Autodesk Inventor part; units mm, degrees
ref_plane "YZ Plane" through (0, 0, 0) normal (1, 0, 0) x (0, 1, 0)
ref_plane "XZ Plane" through (0, 0, 0) normal (0, 1, 0) x (-1, 0, 0)
ref_plane "XY Plane" through (0, 0, 0) normal (0, 0, 1) x (1, 0, 0)
sketch "Эскиз2" plane through (0, 0, 0) normal (0, 0, 1) x (1, 0, 0)
  line L0 (0, 0) -> (12.5, 0)
  line L1 (12.5, 0) -> (12.5, 22.4)
  line L2 (12.5, 22.4) -> (0, 22.4)
  line L3 (0, 22.4) -> (0, 0)
  dimension "d0" = 12.5
  dimension "d1" = 22.4
extrude "Выдавливание1" add sketch "Эскиз2" along normal blind 22.8
sketch "Эскиз3" plane through (0, 22.4, 0) normal (0, 1, 0) x (1, 0, 0)
  line L0 (12.5, 0) -> (0, 0)
  line L1 (12.5, 0) -> (12.5, -18.1)
  line L2 (12.5, 0) -> (12.5, -22.8)
  line L3 (0, 0) -> (0, -22.8)
  line L4 (12.5, -18.1) -> (0, -18.1)
  line L5 (0, -18.1) -> (0, -21.1)
  line L6 (0, -21.1) -> (12.5, -21.1)
  line L7 (12.5, -21.1) -> (12.5, -18.1)
  point P0 (12.5, -21.1)
  point P1 (0, -18.1)
  dimension "d4" = 18.1
  dimension "d5" = 3
extrude "Выдавливание2" add sketch "Эскиз3" along normal blind 4.7 contours L2 L6 L3 L4
sketch "Эскиз4" plane through (0, 0, 0) normal (0, -1, 0) x (1, 0, 0)
  line L0 (12.2114, 0) -> (12.5, 16.0974)
  line L1 (12.5, 0) -> (12.5, 22.8)
  line L2 (12.5, 21.1) -> (12.5, 18.1)
  line L3 (0, 18.1) -> (0, 21.1)
  line L4 (12.5, 18.1) -> (0, 18.1)
  line L5 (0, 18.1) -> (0, 21.1)
  line L6 (0, 21.1) -> (12.5, 21.1)
  line L7 (12.5, 21.1) -> (12.5, 18.1)
  point P0 (0, 0)
  point P1 (12.5, 21.1)
  point P2 (0, 18.1)
  dimension "d8" = 16.1
  dimension "d9" = 3
extrude "Выдавливание3" add sketch "Эскиз4" along normal blind 4.7
sketch "Эскиз5" plane through (0, 0, 21.1) normal (0, 0, 1) x (1, 0, 0)
  line L0 (0, -4.7) -> (12.5, -4.7)
  line L1 (6.25, -4.7) -> (6.25, -2.275)
  line L2 (12.5, 27.1) -> (0, 27.1)
  line L3 (6.25, 27.1) -> (6.25, 24.675)
  circle A0 centre (6.25, -2.275) radius 1
  circle A1 centre (6.25, 24.675) radius 1
  line L4 (6.25, -2.275) -> (7, -2.275)
  line L5 (7, -2.275) -> (7, -4.7)
  line L6 (7, -4.7) -> (6.25, -4.7)
  line L7 (6.25, -4.7) -> (6.25, -2.275)
  line L8 (6.25, -4.7) -> (5.5, -4.7)
  line L9 (5.5, -4.7) -> (5.5, -2.275)
  line L10 (5.5, -2.275) -> (6.25, -2.275)
  line L11 (6.25, -2.275) -> (6.25, -4.7)
  line L12 (6.25, 27.1) -> (7, 27.1)
  line L13 (7, 27.1) -> (7, 24.675)
  line L14 (7, 24.675) -> (6.25, 24.675)
  line L15 (6.25, 24.675) -> (6.25, 27.1)
  line L16 (6.25, 24.675) -> (5.5, 24.675)
  line L17 (5.5, 24.675) -> (5.5, 27.1)
  line L18 (5.5, 27.1) -> (6.25, 27.1)
  line L19 (6.25, 27.1) -> (6.25, 24.675)
  point P0 (0, 0)
  point P1 (5.5, 25.3364)
  point P2 (7, 25.3364)
  point P3 (5.5, -2.9364)
  point P4 (7, -2.9364)
  dimension "d12" = 2.425
  dimension "d13" = 2.425
  dimension "d14" = 2
  dimension "d15" = 2
  dimension "d16" = 0.75
  dimension "d17" = 0.75
  dimension "d18" = 0.75
  dimension "d19" = 0.75
extrude "Выдавливание4" cut sketch "Эскиз5" against normal through all
sketch "Эскиз6" plane through (0, 0, 22.8) normal (0, 0, 1) x (1, 0, 0)
  line L0 (12.5, 0) -> (0, 0)
  line L1 (6.25, 0) -> (6.25, 6.25)
  circle A0 centre (6.25, 6.25) radius 6.25
  line L2 (6.25, 6.25) -> (6.25, 13.5)
  circle A1 centre (6.25, 13.5) radius 2
  point P0 (7.8448, 12.2931)
  dimension "d22" = 6.25
  dimension "d23" = 12.5
  dimension "d24" = 7.25
  dimension "d25" = 4
extrude "Выдавливание5" add sketch "Эскиз6" along normal blind 5
sketch "Эскиз7" plane through (0, 0, 27.8) normal (0, 0, 1) x (1, 0, 0)
  arc A0 (4.6552, 12.2931) -> (0, 6.25) centre (6.25, 6.25) ccw
  circle A1 centre (6.25, 6.25) radius 1.5
  point P0 (0, 0)
  dimension "d28" = 3
extrude "Выдавливание6" add sketch "Эскиз7" along normal blind 4.6
properties part number "Сервопривод SG90"
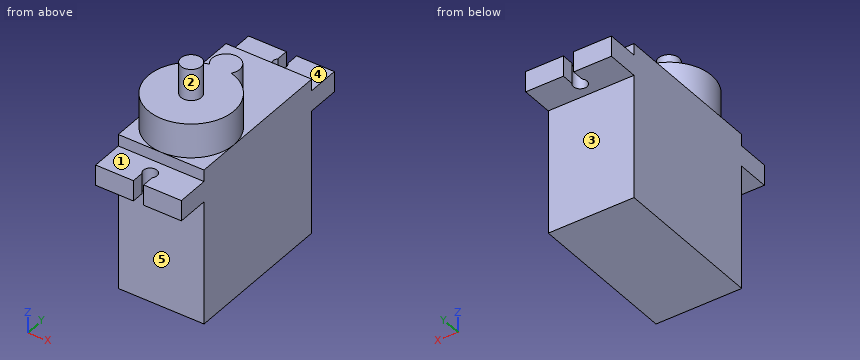
Check sheet for the modelled part. Datum: model origin and axes. Units: mm. Face numbers are marked on the shaded views. A direction names the side the tool comes from. Give positions to 0.01 mm unless a question says otherwise; leave off trailing zeros. Write each loop counter-clockwise with the first axis right and the second up, starting at its lowest first coordinate (ties: lowest second). Pieces come first, ordered by that corner, then holes. Notation, with made-up numbers: (27, 16.5) -> (56, 16.5) arc R25 cw to (56, 30.5) -> close; hole circle Ø5 at (16, -16). An arc over 180 degrees is marked (long way). One line per item, written item: value. Start each with the question number.
Item 1: Tool access check on the marked faces 1, 2, 3, 4 and 5. Record the directions out of +Z, -Z, +X, -X, +Y, -Y that give a thin tool (end or side, any length) a straight path to the whole face; none if there is none.
Item 2: Gauge pin test, flat ends, axial feed: pin 1 (6 mm diameter, centred on x = 4.5, z = 3.5, fed in from +Y); pin 2 (1 mm diameter, centred on x = 7, y = 14, fed in from +Z); pin 3 (3 mm diameter, centred on x = 6.25, y = -2.275, fed in from -Z). Record the tip position at first contact, or that the pin passes through.
Item 3: Material ranges on probe 1 along Y at (x, z) = (2.25, 14); probe 2 along Y at (x, z) = (6.25, 18.9) (3 decimals); probe 3 along Z at (x, y) = (3.75, 25), recorded low to high. Write a range as from..to.
Item 4: Section check D-D on y = 4. Record the cut outline in (x, z).
Item 5: Section check A-A on y = 13.5. Record the cut outline in (x, z), then the cut area to 3 significant figures.
Item 6: Section check C-C on z = 6. Record the cut outline in (x, y).
Item 7: Section check B-B on x = 9. Record the cut outline in (y, z), then the cut area to 3 significant figures.
Results list:
1. face 1: +Z, +X, -X, -Y
1. face 2: +Z
1. face 3: -Z, +X, -X, +Y
1. face 4: +Z, +X, -X, +Y
1. face 5: -Z, +X, -X, -Y
2. pin 1: y = 22.4
2. pin 2: z = 27.8
2. pin 3: z = 18.1
3. probe 1: 0..22.4
3. probe 2: -1.275..23.675
3. probe 3: 18.1..21.1
4. outline: (0, 0) -> (12.5, 0) -> (12.5, 22.8) -> (12.08, 22.8) -> (12.08, 27.8) -> (0.42, 27.8) -> (0.42, 22.8) -> (0, 22.8) -> close
5. outline: (0, 0) -> (12.5, 0) -> (12.5, 22.8) -> (8.25, 22.8) -> (8.25, 27.8) -> (4.25, 27.8) -> (4.25, 22.8) -> (0, 22.8) -> close
5. area: 305 mm²
6. outline: (0, 0) -> (12.5, 0) -> (12.5, 22.4) -> (0, 22.4) -> close
7. outline: (-4.7, 18.1) -> (0, 18.1) -> (0, 0) -> (22.4, 0) -> (22.4, 18.1) -> (27.1, 18.1) -> (27.1, 21.1) -> (22.4, 21.1) -> (22.4, 22.8) -> (11.86, 22.8) -> (11.86, 27.8) -> (0.64, 27.8) -> (0.64, 22.8) -> (0, 22.8) -> (0, 21.1) -> (-4.7, 21.1) -> close
7. area: 595 mm²
